Autodesk Inventor part; units mm, degrees
ref_plane "YZ Plane" through (0, 0, 0) normal (1, 0, 0) x (0, 1, 0)
ref_plane "XZ Plane" through (0, 0, 0) normal (0, 1, 0) x (-1, 0, 0)
ref_plane "XY Plane" through (0, 0, 0) normal (0, 0, 1) x (1, 0, 0)
sketch "Sketch1" plane through (0, 0, 0) normal (1, 0, 0) x (0, 1, 0)
  arc A0 (30.5, -3.2113) -> (29.5, -3.2113) centre (30, 0) ccw
  arc A1 (35, -5.25) -> (32.7265, 6.7178) centre (30, 0) ccw
  line L0 (0, 0) -> (50.3094, 0) construction
  line L1 (0, 20) -> (0, -20)
  line L2 (0, 20) -> (32.7265, 6.7178)
  line L3 (30, 0) -> (30, -135) construction
  line L4 (30.5, -3.2113) -> (30.5, -15.25)
  line L5 (32.5, -5.25) -> (32.5, -15.25)
  line L6 (32.5, -5.25) -> (35, -5.25)
  line L7 (32.5, -15.25) -> (30.5, -15.25)
  line L8 (29.5, -3.2113) -> (29.5, -15.25)
  line L9 (0, -20) -> (29.5, -15.25)
  point P0 (30, -3.25)
  dimension "d1" = 6.5
  dimension "d2" = 30
  dimension "d3" = 14.5
  dimension "d4" = 40
  dimension "d17" = 0.5
  dimension "d18" = 10
  dimension "d19" = 2
  dimension "d20" = 2
  dimension "d21" = 1
  dimension "d24" = 20
extrude "Extrusion1" add sketch "Sketch1" along normal blind 10
sketch "Sketch2" plane through (0, 32.5, -5.25) normal (0, 1, 0) x (1, 0, 0)
  line L0 (5, -5.25) -> (5, 25.2229) construction
  line L1 (0, 10) -> (0, 0) construction
  arc A0 (2.75, 4.25) -> (7.25, 4.25) centre (5, 4.25) ccw
  arc A1 (7.25, 5.75) -> (2.75, 5.75) centre (5, 5.75) ccw
  line L2 (2.75, 4.25) -> (2.75, 5.75)
  line L3 (7.25, 4.25) -> (7.25, 5.75)
  line L4 (0, 10) -> (10, 10)
  line L5 (0, 10) -> (0, 0)
  line L6 (0, 0) -> (10, 0)
  line L7 (10, 10) -> (10, 0)
  line L8 (0, 10) -> (10, 10)
  point P0 (0, -5.25)
  dimension "d27" = 5
  dimension "d28" = 4.5
  dimension "d29" = 4.5
  dimension "d30" = 1.5
  dimension "d31" = 4.25
extrude "Extrusion2" cut sketch "Sketch2" against normal up to surface (2 mm away) contours L2 A1 L3 A0
sketch "Sketch3" plane through (0, 29.5, -3.2113) normal (0, 1, 0) x (1, 0, 0)
  line L0 (2.75, 6.2887) -> (2.75, 7.7887)
  arc A0 (7.25, 7.7887) -> (2.75, 7.7887) centre (5, 7.7887) ccw
  line L1 (7.25, 7.7887) -> (7.25, 6.2887)
  arc A1 (2.75, 6.2887) -> (7.25, 6.2887) centre (5, 6.2887) ccw
  line L2 (0, 12.0387) -> (0, 2.0387)
  line L3 (0, 2.0387) -> (10, 2.0387)
  line L4 (10, 12.0387) -> (10, 2.0387)
  line L5 (0, 12.0387) -> (10, 12.0387)
  circle A2 centre (5, 7.0387) radius 2
  line L6 (5, 6.2887) -> (5, 7.7887)
  point P0 (0, -3.2113)
  dimension "d34" = 4
  dimension "d35" = 1.5
  dimension "d36" = 0.75
extrude "Extrusion3" cut sketch "Sketch3" against normal blind 10 contours A2
equation "\"d17\" = 0.5 * d21"
equation "\"d24\" = 0.5 * d4"
equation "\"d36\" = 0.5 * d35"
properties part number "mocowanie walka"
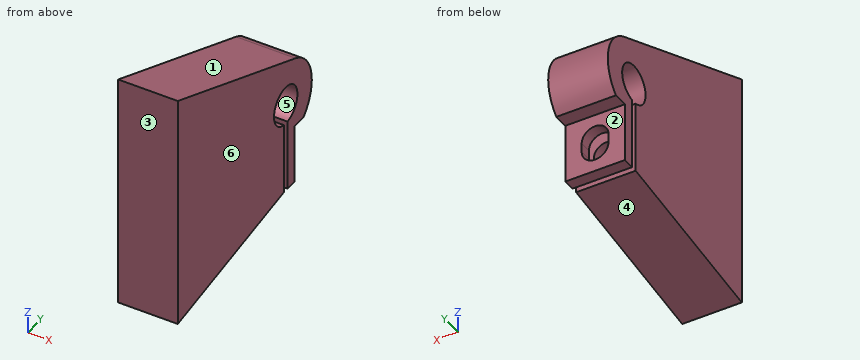
Part model, mm, in its own coordinate system. Face numbers are marked on the shaded views. A direction names the side the tool comes from. Give positions to 0.01 mm unless a question says otherwise; leave off trailing zeros. Order: outer loops, then holes, each group sorted by start corner. A loop starts at its lowest first (then second) coordinate and runs counter-clockwise, first axis right, second up. Notation, with made-up numbers: M 13,54.25 L 33,54.25 A26 ccw 33,86.25 Z; hole C -26,-18.75 d4. An arc over 180 degrees is marked long. Use a Markdown table: item, result. Add a question column.
(1) Probe line 1 along X through (y, z) = (25.75, -10.25); line 2 along Y through (x, z) = (5.75, -13.5); line 3 along Y through (x, z) = (5.5, 0). List the from-to ranges inside material, lowest first. Write a range as [from, to].
(2) Saw through at B-B, the plane x = 5. Give the cut face in (y, z), and give its area (3 significant figures).
(3) Saw through at A-A, the plane z = 0. Give the cut face in (x, y).
(4) Mould opens along Y. For the marked faces 3, 4, 5 and 6 say: +Y half, -Y half, draft (parallel to the pull), parting line (faces both ways), or undercut.
(5) 3-axis set-ups, long thin cutter, end or side, ignore diameter. For the marked faces 1 and 2: which of +Z, -Z, +X, -X, +Y, -Y reach the whole face in a straight line?
(6) Saw through at D-D, the plane x = 1.75. Give the cut face in (y, z).
(7) Drop flat-ended pins along their axis: P1, Ø5, axis at x = 7, z = -10, coming from the +Y side; P2, Ø3, axis at x = 7, y = 6.5, coming from the +Z side; P3, Ø4, axis at y = 30, z = 0, coming from the +X side; P4, Ø3, axis at x = 4.5, y = 33.5, coming from the -Z side. Give the stop position or say it passes through.
(8) Saw through at C-C, the plane z = -10.25. Give the cut face in (x, y), and give its area (3 significant figures).
Answer key:
| question | item | result |
|---|---|---|
| 1 | line 1 | [0, 3], [7, 10] |
| 1 | line 2 | [0, 29.5], [30.5, 32.5] |
| 1 | line 3 | [0, 26.75], [33.25, 37.25] |
| 2 | outline | M 0,-20 L 29.5,-15.25 L 29.5,-12.25 L 19.5,-12.25 L 19.5,-8.25 L 29.5,-8.25 L 29.5,-3.21 A3.25 cw long 30.5,-3.21 L 30.5,-7.25 L 32.5,-7.25 L 32.5,-5.25 L 35,-5.25 A7.25 ccw 32.73,6.72 L 0,20 Z; M 30.5,-15.25 L 32.5,-15.25 L 32.5,-13.25 L 30.5,-13.25 Z |
| 2 | area | 949 mm^2 |
| 3 | outline | M 0,0 L 10,0 L 10,26.75 L 0,26.75 Z; M 0,33.25 L 10,33.25 L 10,37.25 L 0,37.25 Z |
| 4 | face 3 | -Y half |
| 4 | face 4 | +Y half |
| 4 | face 5 | undercut |
| 4 | face 6 | draft |
| 5 | face 1 | +Z, +X, -X, +Y |
| 5 | face 2 | -Z, +X, -X, +Y |
| 6 | outline | M 0,-20 L 29.5,-15.25 L 29.5,-3.21 A3.25 cw long 30.5,-3.21 L 30.5,-15.25 L 32.5,-15.25 L 32.5,-5.25 L 35,-5.25 A7.25 ccw 32.73,6.72 L 0,20 Z |
| 7 | P1 | y = 32.5 |
| 7 | P2 | z = 17.97 |
| 7 | P3 | through |
| 7 | P4 | z = -15.25 |
| 8 | outline | M 0,0 L 10,0 L 10,29.5 L 7,29.5 L 7,19.5 L 3,19.5 L 3,29.5 L 0,29.5 Z; M 0,30.5 L 2.75,30.5 L 2.75,32.5 L 0,32.5 Z; M 7.25,30.5 L 10,30.5 L 10,32.5 L 7.25,32.5 Z |
| 8 | area | 266 mm^2 |
